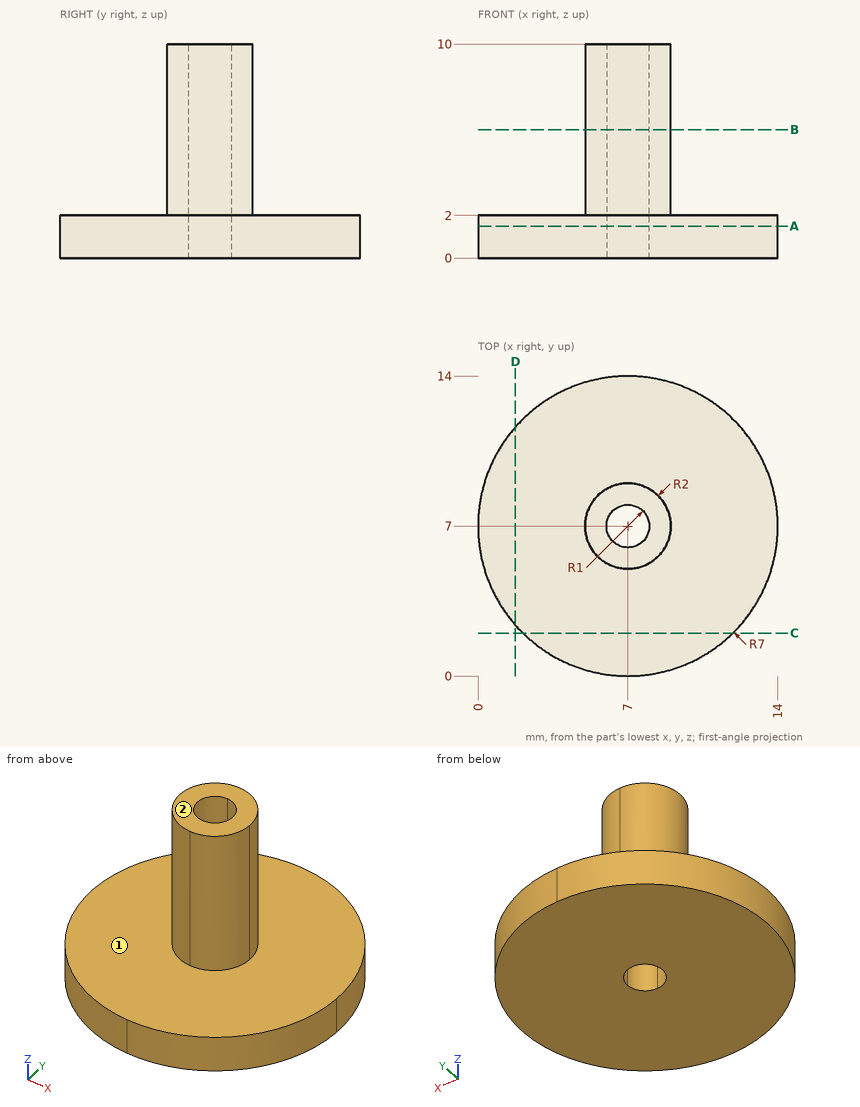
Study the drawing (mm; zero at the part's minimum x, y, z) and answer. A direction names the side the tool comes from. Give positions to 0.01 mm unless a question says otherwise; leave off trailing zeros. Loops run counter-clockwise (first coordinate to the right, second up) from the corner with the lowest first, then second, coordinate; pieces in that order, holes last. Notation, with made-up numbers: (72, 64.5) - (111, 64.5) arc R13 ccw to (111, 82.5) - close; hole circle Ø4 at (39, 35). An arc over 180 degrees is marked (long way). Use CSV: the item, a comma, the result in double quotes. Start each with the question number.
(1) Find section C-C, the plane y = 2. Determine the outline of the cut face in (x, z), plus the area to 3 significant figures.
(2) Find the intervals of material crossed by L1, parallel to Y at x = 7, z = 6.5; L2, parallel to Z at x = 6, y = 12; L3, parallel to X at y = 7.25, z = 4.75, in increasing order.
(3) Find section B-B, the plane z = 6. Determine the outline of the cut face in (x, y), plus the area to 3 significant figures.
(4) Find section A-A, the plane z = 1.5. Determine the outline of the cut face in (x, y), plus the area to 3 significant figures.
(5) A tool of negligible diameter and unlimited length cuts with its end or side. For the marked faces 1 and 2, from which of +Z, -Z, +X, -X, +Y, -Y can it reach the whole face along a straight path? Write none if from no direction.
(6) Each of these flat-tipped pins is pushed along its axis until it touches: pin 1 (5 mm diameter, centred on y = 11, z = 1.5, fed in from -X); pin 2 (5 mm diameter, centred on x = 6.5, z = 8, fed in from +Y); pin 3 (1.5 mm diameter, centred on x = 8, z = 1.5, fed in from +Y). Where does it stop, or does it pass through?
(7) Find section D-D, the plane x = 1.75. Determine the outline of the cut face in (y, z).
Results found:
1,outline,"(2.1, 0) - (11.9, 0) - (11.9, 2) - (2.1, 2) - close"
1,area,"19.6 mm^2"
2,L1,"5 to 6, 8 to 9"
2,L2,"0 to 2"
2,L3,"5.02 to 6.03, 7.97 to 8.98"
3,outline,"(7, 5) arc R2 ccw to (9, 7) arc R2 ccw to (7, 9) arc R2 ccw to start; hole (7, 8) arc R1 ccw (long way) to (8, 7) arc R1 ccw to start"
3,area,"9.42 mm^2"
4,outline,"(7, 0) arc R7 ccw to (14, 7) arc R7 ccw to (7, 14) arc R7 ccw to start; hole (7, 8) arc R1 ccw (long way) to (8, 7) arc R1 ccw to start"
4,area,"151 mm^2"
5,face 1,"+Z"
5,face 2,"+Z, +X, -X, +Y, -Y"
6,pin 1,"x = 0.16"
6,pin 2,"y = 9"
6,pin 3,"y = 14"
7,outline,"(2.37, 0) - (11.63, 0) - (11.63, 2) - (2.37, 2) - close"
